Part print with two shaded views. Sizes in mm from the minimum x, y, z corner. A direction names the side the tool comes from. Coordinates: 2 decimals unless noted, no trailing zeros. Loops run counter-clockwise (first coordinate to the right, second up) from the corner with the lowest first, then second, coordinate; pieces in that order, holes last. Notation, with made-up numbers: M 85.5,89.25 L 128.5,89.25 A10 cw 128.5,96.25 Z; hole C 86.25,57 d6. An arc over 180 degrees is marked long. Use CSV: the item, a comma, the result in double quotes. Start each with the question number.
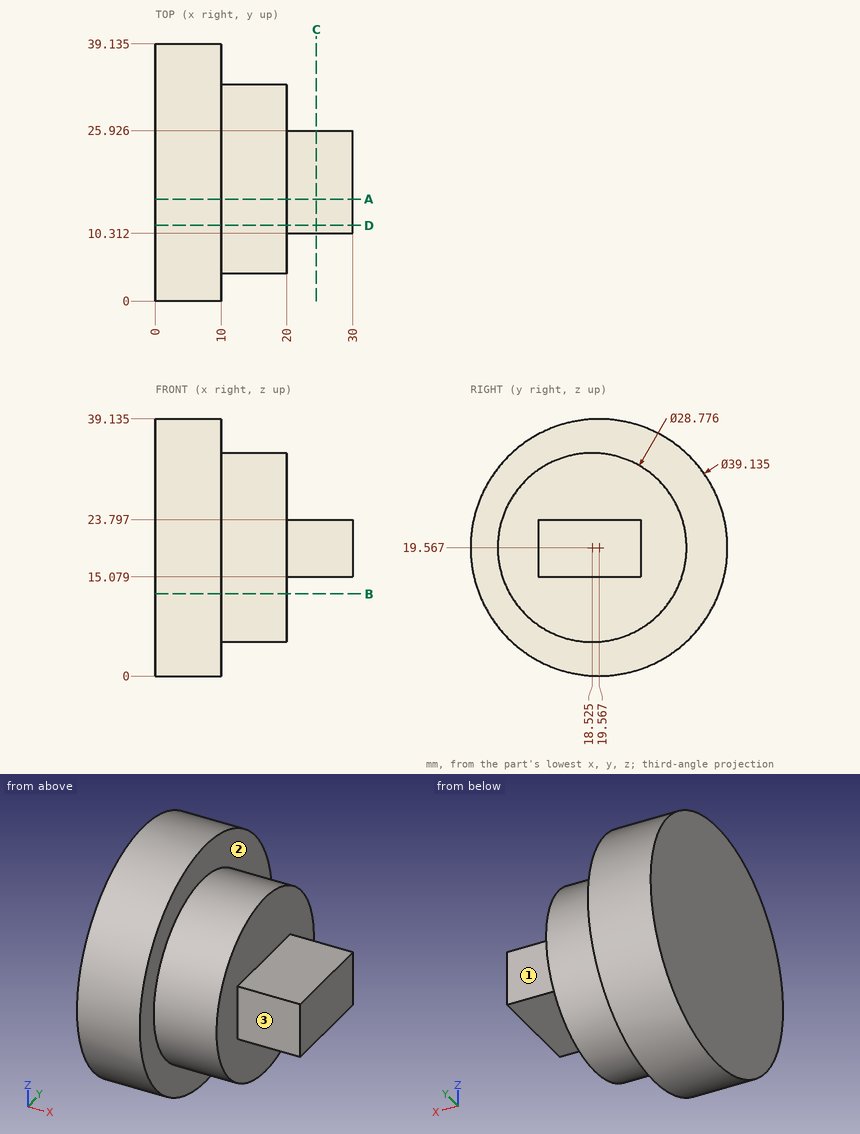
1. Tool access for the marked faces 1, 2 and 3: list every direction of +Z, -Z, +X, -X, +Y, -Y with a clear straight run to the whole face (end or side of a thin tool).
2. Wall check: probe 1 along X at (y, z) = (18.5, 29.5); probe 2 along X at (y, z) = (33, 15); probe 3 along Z at (x, y) = (21.75, 10.5). Give the ranges that are in metal, low to high.
3. Slice it at D-D, the plane y = 11.5. List the corners of the cut face in (x, z) (1 decimal).
4. Pin check, flat tips, straight feed: pin 1 (9.5 mm diameter, centred on x = 26, z = 19, fed in from +Y); pin 2 (2.5 mm diameter, centred on x = 24, z = 20, fed in from -Y); pin 3 (8 mm diameter, centred on x = 23.5, y = 20.5, fed in from -Z). Stop position of each tip, or through.
5. Slice it at A-A, the plane y = 15.5. List the corners of the cut face in (x, z).
6. Slice it at B-B, the plane z = 12.5. List the corners of the cut face in (x, y).
7. Slice it at C-C, the plane x = 24.5. List the corners of the cut face in (y, z).
Found:
1,face 1,"+Z, -Z, +X, +Y"
1,face 2,"+X"
1,face 3,"+Z, -Z, +X, -Y"
2,probe 1,"0 to 20"
2,probe 2,"0 to 10"
2,probe 3,"15.08 to 23.8"
3,outline,"M 0,1.7 L 10,1.7 L 10,7 L 20,7 L 20,15.1 L 30,15.1 L 30,23.8 L 20,23.8 L 20,32.1 L 10,32.1 L 10,37.4 L 0,37.4 Z"
4,pin 1,"y = 25.93"
4,pin 2,"y = 10.31"
4,pin 3,"z = 5.18"
5,outline,"M 0,0.43 L 10,0.43 L 10,5.5 L 20,5.5 L 20,15.08 L 30,15.08 L 30,23.8 L 20,23.8 L 20,33.63 L 10,33.63 L 10,38.71 L 0,38.71 Z"
6,outline,"M 0,1.32 L 10,1.32 L 10,5.99 L 20,5.99 L 20,31.06 L 10,31.06 L 10,37.81 L 0,37.81 Z"
7,outline,"M 10.31,15.08 L 25.93,15.08 L 25.93,23.8 L 10.31,23.8 Z"
